Design review of the part built by this model. Coordinates are the model's own, in mm. A direction names the side the tool comes from. Coordinates: 2 decimals unless noted, no trailing zeros. Order: outer loops, then holes, each group sorted by start corner. A loop starts at its lowest first (then second) coordinate and runs counter-clockwise, first axis right, second up. Notation, with made-up numbers: M 28,77.25 L 65,77.25 A16 cw 65,107.25 Z; hole C -24.75,16.25 d7. An arc over 180 degrees is marked long. Answer as a JSON object with one key per item and string values.
Autodesk Inventor part; units mm, degrees
ref_plane "YZ Plane" through (0, 0, 0) normal (1, 0, 0) x (0, 1, 0)
ref_plane "XZ Plane" through (0, 0, 0) normal (0, 1, 0) x (-1, 0, 0)
ref_plane "XY Plane" through (0, 0, 0) normal (0, 0, 1) x (1, 0, 0)
sketch "Sketch1" plane through (0, 0, 0) normal (0, 1, 0) x (-1, 0, 0)
  circle A0 centre (0, 0) radius 3.4
  dimension "d3" = 6.8
extrude "Extrusion1" add sketch "Sketch1" along normal blind 3.75
sketch "Sketch2" plane through (0, 0, 0) normal (0, -1, 0) x (1, 0, 0)
  circle A0 centre (0, 0) radius 2.3583
extrude "Extrusion2" cut sketch "Sketch2" against normal blind 2.25
sketch "Sketch3" plane through (0, 3.75, 0) normal (0, 1, 0) x (1, 0, 0)
  circle A0 centre (0, 0) radius 3.4 construction
  line L0 (0, -3.4) -> (0, 3.4) construction
  circle A1 centre (-11.85, 0.0077) radius 2
  line L1 (-12.0876, -1.9781) -> (-0.4039, -3.3759)
  line L2 (-12.085, 1.9939) -> (-0.3995, 3.3764)
  circle A2 centre (0, 0) radius 3.4
  dimension "d6" = 4
  dimension "d7" = 11.85
extrude "Extrusion3" add sketch "Sketch3" against normal blind 2.1 contours A1 | A1 L2 A2 L1
mirror "Mirror1" about plane through (0, 0, 0) normal (1, 0, 0) of "Extrusion3"
sketch "Sketch4" plane through (0, 3.75, 0) normal (0, 1, 0) x (1, 0, 0)
  circle A0 centre (12.2999, 0) radius 0.55
  arc A1 (12.0876, -1.9781) -> (12.085, 1.9939) centre (11.85, 0.0077) ccw
  line L0 (0, 0) -> (13.85, 0) construction
  circle A2 centre (10.2999, 0) radius 0.55
  circle A3 centre (8.2999, 0) radius 0.55
  circle A4 centre (6.2999, 0) radius 0.55
  circle A5 centre (4.2999, 0) radius 0.55
  dimension "d10" = 1.1
  dimension "d11" = 1
  dimension "d14" = 2
extrude "Extrusion4" cut sketch "Sketch4" against normal blind 2.1
mirror "Mirror2" about plane through (0, 0, 0) normal (1, 0, 0) of "Extrusion4"
properties part number "stick"
1) Add section C-C (z = -1.25). State the section outline as (x, y) points.
Taken from the geometry:
{"outline": "M -13.42,1.65 L -3.16,1.65 L -3.16,0 L -2,0 L -2,2.25 L 2,2.25 L 2,0 L 3.16,0 L 3.16,1.65 L 13.42,1.65 L 13.42,3.75 L -13.42,3.75 Z"}
2) Tool access review of faces 4 (the cylindrical face through (0.44, 0.6, -3.37)), 5 (the cylindrical face through (-3.75, 2.71, 0.02)): name each direction out of +Z, -Z, +X, -X, +Y, -Y from which nothing blocks a thin tool from reaching the whole face with its end or side.
Taken from the geometry:
{"face 4": "-Y", "face 5": "+Y, -Y"}
3) Mouldability with a two-part tool opening along Z and no side actions: class faces 1 (the flat face through (6.164, 2.715, 2.687)), 2 (the flat face through (-7, 1.65, 0)), 3 (the flat face through (0, 2.25, 0)) as released by +Z, released by -Z, zero draft, split by the parting line, or undercut.
Taken from the geometry:
{"face 1": "released by +Z", "face 2": "zero draft", "face 3": "undercut"}
4) Insertion check: pin 1 Ø1.5 at (y, z) = (2.5, -0.5) entering from -X; pin 2 Ø0.9 at (x, z) = (6.3, 0) entering from +Y; pin 3 Ø4 at (x, z) = (0, 0) entering from -Y; pin 4 Ø1.8 at (x, z) = (-6.3, 0) entering from -Y. Each pin has a flat end and moves straight along its axis. Give the tip position at first contact, or say it passes through.
Taken from the geometry:
{"pin 1": "stops at x = -13.85", "pin 2": "passes through", "pin 3": "stops at y = 2.25", "pin 4": "stops at y = 1.65"}
5) Add section D-D (x = 0). State the section outline as (y, z) points.
Taken from the geometry:
{"outline": "M 0,-3.4 L 3.75,-3.4 L 3.75,3.4 L 0,3.4 L 0,2.36 L 2.25,2.36 L 2.25,-2.36 L 0,-2.36 Z"}
6) Add section A-A (x = 4). State the section outline as (y, z) points.
Taken from the geometry:
{"outline": "M 1.65,-2.95 L 3.75,-2.95 L 3.75,-0.46 L 1.65,-0.46 Z; M 1.65,0.46 L 3.75,0.46 L 3.75,2.95 L 1.65,2.95 Z"}
7) Add section B-B (y = 0.75). State the section outline as (x, z) points.
Taken from the geometry:
{"outline": "C 0,0 d6.8; hole C 0,0 d4.72"}
8) To check wall thickness, follow L1, parallel to Z at x = 8.25, y = 2.35; L2, parallel to Z at x = 10.75, y = 2.3; L3, parallel to Y at x = -0.25, z = -1.5. State the ranges of each line that lie inside material, in increasing order.
Taken from the geometry:
{"L1": "z = -2.45 to -0.55, 0.55 to 2.44", "L2": "z = -2.15 to -0.32, 0.32 to 2.14", "L3": "y = 2.25 to 3.75"}
